Autodesk Inventor part; units mm, degrees
ref_plane "YZ Plane" through (0, 0, 0) normal (1, 0, 0) x (0, 1, 0)
ref_plane "XZ Plane" through (0, 0, 0) normal (0, 1, 0) x (-1, 0, 0)
ref_plane "XY Plane" through (0, 0, 0) normal (0, 0, 1) x (1, 0, 0)
sketch "Sketch4" plane through (0, 0, 0) normal (0, 0, 1) x (1, 0, 0)
  line L0 (0, 0) -> (0, 8)
  line L1 (0, 8) -> (51.5, 8)
  line L2 (51.5, 8) -> (51.5, 16.65)
  line L3 (51.5, 16.65) -> (56.5, 23.25)
  line L4 (56.5, 23.25) -> (56.5, 75)
  arc A0 (101.5, 75) -> (56.5, 75) centre (79, 54.6875) ccw
  line L5 (101.5, 75) -> (101.5, 60)
  line L6 (101.5, 60) -> (114, 52)
  line L7 (114, 52) -> (114, 0)
  line L8 (114, 0) -> (0, 0)
  line L9 (101.5, 75) -> (56.5, 75)
  point P0 (79, 75)
  dimension "d6" = 8
  dimension "d7" = 16.65
  dimension "d8" = 23.25
  dimension "d9" = 75
  dimension "d10" = 85
  dimension "d11" = 15
  dimension "d12" = 8
  dimension "d13" = 51.5
  dimension "d14" = 5
  dimension "d15" = 45
  dimension "d16" = 12.5
revolve "Revolution1" add sketch "Sketch4" angle 360 about axis through (114, 0, 0) along (-1, 0, 0)
sketch "Sketch5" plane through (0, 0, 0) normal (-1, 0, 0) x (0, 0, 1)
  line L0 (-5.3, -5.9925) -> (-5.3, 5.9925)
  circle A0 centre (0, 0) radius 8
  circle A1 centre (0, 0) radius 8
  arc A2 (-5.3, 5.9925) -> (-5.3, -5.9925) centre (0, 0) ccw
  point P0 (0, 0)
  point P1 (-8, 0)
  dimension "d18" = 5.3
extrude "Extrusion3" cut sketch "Sketch5" against normal blind 46.5 contours A0 L0 picked at (-6.6076, -0.8031)
sketch "Sketch6" plane through (0, 0, 0) normal (-1, 0, 0) x (0, 0, 1)
  circle A0 centre (0, 0) radius 8
  line L0 (-5.3, -5.9925) -> (-5.3, 5.9925)
  arc A1 (-5.3, 5.9925) -> (-5.3, -5.9925) centre (0, 0) ccw
  point P0 (0, 0)
  point P1 (-8, 0)
extrude "Extrusion4" add sketch "Sketch6" against normal blind 2.5
sketch "Sketch7" plane through (0, 0, 0) normal (-1, 0, 0) x (0, 0, 1)
  circle A0 centre (0, 0) radius 3.75
  point P0 (0, 0)
  dimension "d23" = 7.5
extrude "Extrusion5" cut sketch "Sketch7" against normal up to surface (56.5 mm away)
properties part number "Wheel" material "Stainless Steel"
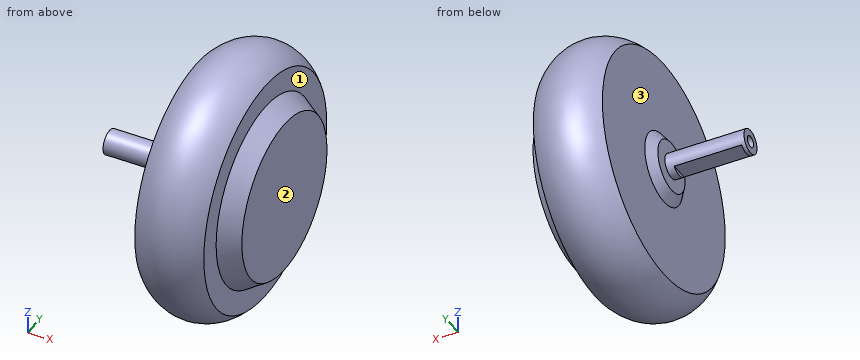
Geometry check sheet. Reference: the model listing, model coordinates, mm. Face numbers are marked on the shaded views. A direction names the side the tool comes from. Coordinates: 2 decimals unless noted, no trailing zeros. Order: outer loops, then holes, each group sorted by start corner. A loop starts at its lowest first (then second) coordinate and runs counter-clockwise, first axis right, second up. Notation, with made-up numbers: (10, 20.25) - (37, 20.25) arc R23 ccw to (37, 32.25) - close; hole circle Ø10 at (6.5, 61). An arc over 180 degrees is marked (long way). Answer in a Markdown table with one row per item. Add a question column.
1. Gauge pin test, flat ends, axial feed: pin 1 Ø8 at (x, z) = (69.5, 9) entering from +Y; pin 2 Ø6 at (x, y) = (30.5, 2.5) entering from -Z; pin 3 Ø4 at (y, z) = (-67, -7) entering from +X. Record the tip position at first contact, or that the pin passes through.
2. Section check C-C (x = 12.5). Enter the section's corners in (y, z).
3. Section check D-D (x = 91). Enter the section's corners in (y, z).
4. Access from +Z, -Z, +X, -X, +Y, -Y to the whole of each face (thin tool, end or side, straight path). Record for the marked faces 1, 2 and 3.
5. Material ranges on L1, parallel to Y at x = 26, z = 0; L2, parallel to Z at x = 39, y = 1; L3, parallel to X at y = -24.5, z = -35, recorded low to high. Write a range as [from, to].
Data:
| question | item | result |
|---|---|---|
| 1 | pin 1 | stops at y = 84.11 |
| 1 | pin 2 | stops at z = -5.3 |
| 1 | pin 3 | stops at x = 101.5 |
| 2 | outline | (-5.99, -5.3) - (5.99, -5.3) arc R8 ccw (long way) to start; hole circle Ø7.5 at (0, 0) |
| 3 | outline | circle Ø165.05 at (0, 0) |
| 4 | face 1 | +X |
| 4 | face 2 | +Z, -Z, +X, +Y, -Y |
| 4 | face 3 | -X |
| 5 | L1 | y = [-8, -3.75], [3.75, 8] |
| 5 | L2 | z = [-5.3, -3.61], [3.61, 7.94] |
| 5 | L3 | x = [56.5, 114] |
